```python
from build123d import *

# Parameters (mm, degrees)
F0_W     = 4.6228
F0_H     = 4.6228
F1_DEPTH = 3.175


with BuildPart() as f1:
    # F0 (on Front) → F1 (new body)
    with BuildSketch(Plane.XZ):
        Polygon((-2.011181, 18.956908), (-41.698681, 18.956908), (-41.698681, -31.843092), (37.676319, -31.843092), (37.676319, 18.956908), align=None)
        with Locations((-35.348681, -25.493092)):
            Rectangle(F0_W, F0_H, mode=Mode.SUBTRACT)
        with Locations((-22.648681, -25.493092)):
            Rectangle(F0_W, F0_H, mode=Mode.SUBTRACT)
        with Locations((-9.948681, -25.493092)):
            Rectangle(F0_W, F0_H, mode=Mode.SUBTRACT)
        with Locations((-35.348681, -12.793092)):
            Rectangle(F0_W, F0_H, mode=Mode.SUBTRACT)
        with Locations((-22.648681, -12.793092)):
            Rectangle(F0_W, F0_H, mode=Mode.SUBTRACT)
        with Locations((-9.948681, -12.793092)):
            Rectangle(F0_W, F0_H, mode=Mode.SUBTRACT)
        with Locations((5.926319, -25.493092)):
            Rectangle(F0_W, F0_H, mode=Mode.SUBTRACT)
        with Locations((18.626319, -25.493092)):
            Rectangle(F0_W, F0_H, mode=Mode.SUBTRACT)
        with Locations((31.326319, -25.493092)):
            Rectangle(F0_W, F0_H, mode=Mode.SUBTRACT)
        with Locations((5.926319, -12.793092)):
            Rectangle(F0_W, F0_H, mode=Mode.SUBTRACT)
        with Locations((18.626319, -12.793092)):
            Rectangle(F0_W, F0_H, mode=Mode.SUBTRACT)
        with Locations((31.326319, -12.793092)):
            Rectangle(F0_W, F0_H, mode=Mode.SUBTRACT)
        with Locations((-35.348681, -0.093092)):
            Rectangle(F0_W, F0_H, mode=Mode.SUBTRACT)
        with Locations((-22.648681, -0.093092)):
            Rectangle(F0_W, F0_H, mode=Mode.SUBTRACT)
        with Locations((-9.948681, -0.093092)):
            Rectangle(F0_W, F0_H, mode=Mode.SUBTRACT)
        with Locations((-35.348681, 12.606908)):
            Rectangle(F0_W, F0_H, mode=Mode.SUBTRACT)
        with Locations((-22.648681, 12.606908)):
            Rectangle(F0_W, F0_H, mode=Mode.SUBTRACT)
        with Locations((-9.948681, 12.606908)):
            Rectangle(F0_W, F0_H, mode=Mode.SUBTRACT)
        with Locations((5.926319, -0.093092)):
            Rectangle(F0_W, F0_H, mode=Mode.SUBTRACT)
        with Locations((18.626319, -0.093092)):
            Rectangle(F0_W, F0_H, mode=Mode.SUBTRACT)
        with Locations((31.326319, -0.093092)):
            Rectangle(F0_W, F0_H, mode=Mode.SUBTRACT)
        with Locations((5.926319, 12.606908)):
            Rectangle(F0_W, F0_H, mode=Mode.SUBTRACT)
        with Locations((18.626319, 12.606908)):
            Rectangle(F0_W, F0_H, mode=Mode.SUBTRACT)
        with Locations((31.326319, 12.606908)):
            Rectangle(F0_W, F0_H, mode=Mode.SUBTRACT)
    extrude(amount=F1_DEPTH)


solid = f1.part
```
Here's how the part is built. I have some questions about the finished solid (model axes, mm). Round coordinates to 2 decimals unless told otherwise and drop trailing zeros. Order: outer loops, then holes, each group sorted by start corner. A loop starts at its lowest first (then second) coordinate and runs counter-clockwise, first axis right, second up. Notation, with made-up numbers: M 22,33.25 L 57,33.25 A26 ccw 57,71.25 Z; hole C 40.5,-34 d3. An arc over 180 degrees is marked long. Answer as CSV lines item,"result".
Item 1: Imagine slicing it at C-C on y = -0.6. Give the number of separate pieces and of enclosed holes in the cut face, and give its area (3 significant figures).
From the geometry:
separate pieces,"1"
enclosed holes,"24"
area,"3,520 mm2"
Item 2: We'd pull the mould along X, two halves only. Please class faces 1 (the flat face through (-41.699, -2, -6)), 2 (the flat face through (-10, -2, -10.482)), 3 (the flat face through (-1, -2, 18.957)): +X half, -X half, draft (parallel to the pull), parting line (faces both ways), or undercut.
From the geometry:
face 1,"-X half"
face 2,"undercut"
face 3,"draft"
Item 3: Please list where this line runs through material, in increasing order: L1, parallel to Z at x = 16.5, y = -0.5. Write a range as [from, to].
From the geometry:
L1,"[-31.84, -27.8], [-23.18, -15.1], [-10.48, -2.4], [2.22, 10.3], [14.92, 18.96]"
Item 4: Imagine slicing it at A-A on z = -12.5. List the corners of the cut face in (x, y) for me (3 decimals).
From the geometry:
outline,"M -41.699,-3.175 L -37.66,-3.175 L -37.66,0 L -41.699,0 Z; M -33.037,-3.175 L -24.96,-3.175 L -24.96,0 L -33.037,0 Z; M -20.337,-3.175 L -12.26,-3.175 L -12.26,0 L -20.337,0 Z; M -7.637,-3.175 L 3.615,-3.175 L 3.615,0 L -7.637,0 Z; M 8.238,-3.175 L 16.315,-3.175 L 16.315,0 L 8.238,0 Z; M 20.938,-3.175 L 29.015,-3.175 L 29.015,0 L 20.938,0 Z; M 33.638,-3.175 L 37.676,-3.175 L 37.676,0 L 33.638,0 Z"
Item 5: Imagine slicing it at B-B on x = 7. List the corners of the cut face in (y, z) for me (1 decimal).
From the geometry:
outline,"M -3.2,-31.8 L 0,-31.8 L 0,-27.8 L -3.2,-27.8 Z; M -3.2,-23.2 L 0,-23.2 L 0,-15.1 L -3.2,-15.1 Z; M -3.2,-10.5 L 0,-10.5 L 0,-2.4 L -3.2,-2.4 Z; M -3.2,2.2 L 0,2.2 L 0,10.3 L -3.2,10.3 Z; M -3.2,14.9 L 0,14.9 L 0,19 L -3.2,19 Z"
